Part print with two shaded views. Sizes in mm from the minimum x, y, z corner. A direction names the side the tool comes from. Give positions to 0.01 mm unless a question says otherwise; leave off trailing zeros. Loops run counter-clockwise (first coordinate to the right, second up) from the corner with the lowest first, then second, coordinate; pieces in that order, holes last. Notation, with made-up numbers: M 22.5,24.5 L 32.5,24.5 A33 ccw 32.5,55.5 Z; hole C 87,8.25 d6. An arc over 180 degrees is marked long. Answer as a JSON object with one key per item and string values. Group by question number.
1. Slice it at B-B (z = 31). List the corners of the cut face in (x, y), then the cut area to 3 significant figures.
2. Slice it at A-A (x = 36). List the corners of the cut face in (y, z) (1 decimal).
3. 3-axis set-ups, long thin cutter, end or side, ignore diameter. For the marked faces 4 and 5: which of +Z, -Z, +X, -X, +Y, -Y reach the whole face in a straight line?
4. Slice it at D-D (x = 58). List the corners of the cut face in (y, z) (1 decimal).
5. Slice it at C-C (x = 44.5). List the corners of the cut face in (y, z) (1 decimal).
6. Drop flat-ended pins along their axis: pin 1 Ø1 at (x, y) = (8, 5.5) entering from -Z; pin 2 Ø2 at (x, y) = (10.5, 4.5) entering from -Z; pin 3 Ø2 at (x, y) = (54.5, 1) entering from +Z. Give the stop position or say it passes through.
7. Drill centre lines: line 1 along X through (y, z) = (4.75, 32.5); line 2 along Z through (x, y) = (17.5, 2.25) (1 decimal); line 3 along Z through (x, y) = (32, 4.75) (1 decimal). Where is each one in solid material? Low to high. Write a range as [from, to].
8. Mould opens along X. For the marked faces 1, 2 and 3 say: released by +X, released by -X, zero draft, split by the parting line, or undercut.
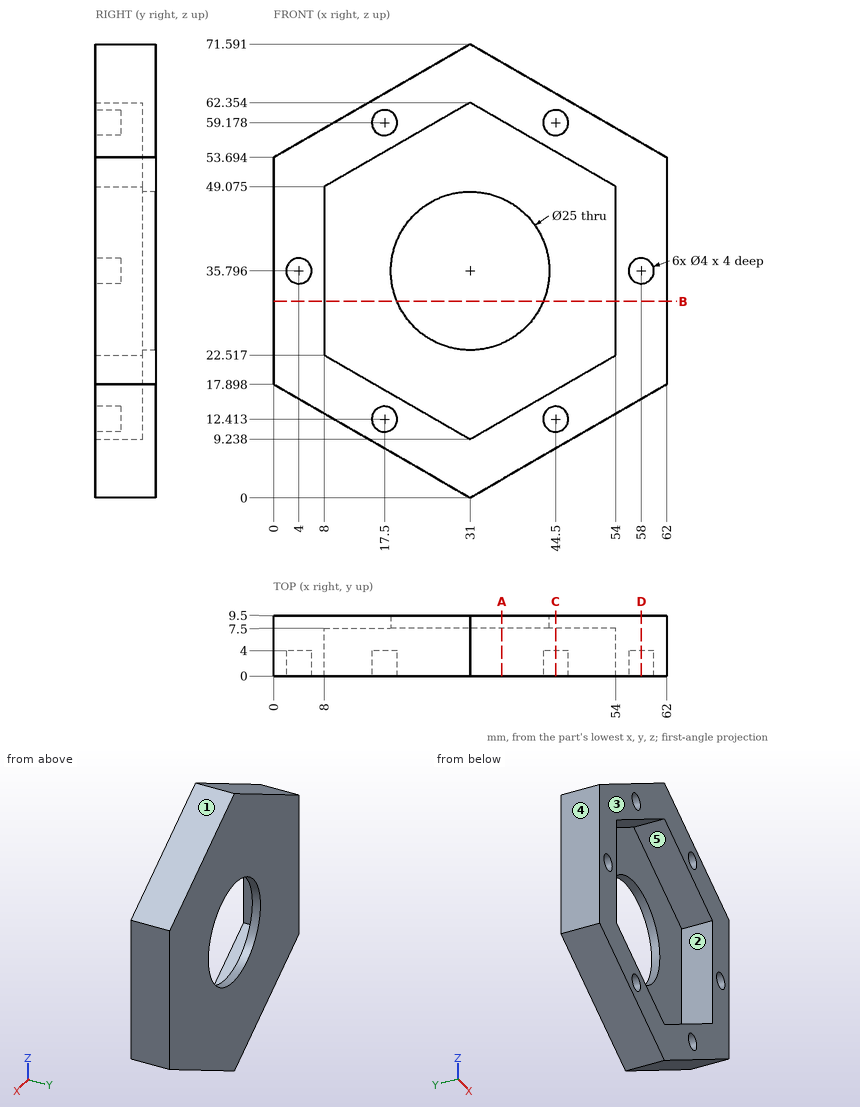
Established:
{
 "1": {"outline": "M 0,0 L 8,0 L 8,7.5 L 19.46,7.5 L 19.46,9.5 L 0,9.5 Z; M 42.54,7.5 L 54,7.5 L 54,0 L 62,0 L 62,9.5 L 42.54,9.5 Z", "area": "198 mm^2"},
 "2": {"outline": "M 0,2.9 L 9.5,2.9 L 9.5,24.3 L 7.5,24.3 L 7.5,12.1 L 0,12.1 Z; M 0,59.5 L 7.5,59.5 L 7.5,47.3 L 9.5,47.3 L 9.5,68.7 L 0,68.7 Z"},
 "3": {"face 4": "+Z, -Z, -X, +Y, -Y", "face 5": "-Y"},
 "4": {"outline": "M 0,15.6 L 9.5,15.6 L 9.5,56 L 0,56 L 0,37.8 L 4,37.8 L 4,33.8 L 0,33.8 Z"},
 "5": {"outline": "M 0,7.8 L 9.5,7.8 L 9.5,63.8 L 0,63.8 L 0,61.2 L 4,61.2 L 4,57.2 L 0,57.2 L 0,54.6 L 7.5,54.6 L 7.5,17 L 0,17 L 0,14.4 L 4,14.4 L 4,10.4 L 0,10.4 Z"},
 "6": {"pin 1": "stops at z = 12.99", "pin 2": "stops at z = 11.26", "pin 3": "stops at z = 58.6"},
 "7": {"line 1": "x = [0, 8], [54, 62]", "line 2": "z = [7.8, 10.4], [14.4, 17], [54.6, 57.2], [61.2, 63.8]", "line 3": "z = [0.6, 9.8], [61.8, 71]"},
 "8": {"face 1": "released by +X", "face 2": "undercut", "face 3": "zero draft"}
}
